from build123d import *

# Parameters (mm, degrees)
SKETCH1_R           = 10.75
BOSS_EXTRUDE1_DEPTH = 3
SKETCH2_R           = 10.75
BOSS_EXTRUDE2_DEPTH = 5.5
DRAFT5_START        = -9.337185289
DRAFT5_DEPTH        = 18.674370578
SKETCH3_W           = 5.126913696
SKETCH3_H           = 18.674370578
BOSS_EXTRUDE3_DEPTH = 17
CUT_EXTRUDE1_REACH  = 59.708
CUT_EXTRUDE2_REACH  = 59.708
SKETCH5_R           = 4


# Read off the part's stored shape, not the designer's step: Draft5
with BuildPart() as part:
    # Sketch1 → Boss-Extrude1 (new body)
    with BuildSketch(Plane(origin=(0, 0, 0), x_dir=(0, 0, -1), z_dir=(1, 0, 0))):
        with BuildLine():
            ThreePointArc((-4.479326664, 23.069148936), (0, -23.5), (4.479326664, 23.069148936))
            ThreePointArc((4.479326664, 23.069148936), (0, 19), (-4.479326664, 23.069148936))
        make_face()
        Circle(SKETCH1_R, mode=Mode.SUBTRACT)
    extrude(amount=BOSS_EXTRUDE1_DEPTH)

    # Sketch2 → Boss-Extrude2 (add)
    # profile 1 of 7: a face of its own
    with BuildSketch(Plane(origin=(3, 0, 0), x_dir=(0, 0, -1), z_dir=(1, 0, 0))):
        with BuildLine():
            Line((-15.626913696, -9.337185289), (-15.626913696, 9.337185289))
            Line((-15.626913696, 9.337185289), (-21.565411447, 9.337185289))
            ThreePointArc((-21.565411447, 9.337185289), (-22.146716975, 7.859575512), (-22.626913696, 6.346083564))
            Line((-22.626913696, 6.346083564), (-22.626913696, -6.346083564))
            ThreePointArc((-22.626913696, -6.346083564), (-22.146716975, -7.859575512), (-21.565411447, -9.337185289))
            Line((-21.565411447, -9.337185289), (-15.626913696, -9.337185289))
        make_face()
    # profile 2 of 7: a face of its own
    with BuildSketch(Plane(origin=(3, 0, 0), x_dir=(0, 0, -1), z_dir=(1, 0, 0))):
        Polygon((-15.626913696, -9.337185289), (-15.626913696, 9.337185289), (-8.736803998, 14.760144229), (8.736803998, 14.760144229), (15.626913696, 9.337185289), (15.626913696, -9.337185289), (8.736803998, -14.760144229), (-8.736803998, -14.760144229), align=None)
        Circle(SKETCH2_R, mode=Mode.SUBTRACT)
    # profile 3 of 7: a face of its own
    with BuildSketch(Plane(origin=(3, 0, 0), x_dir=(0, 0, -1), z_dir=(1, 0, 0))):
        with BuildLine():
            Line((21.565411447, 9.337185289), (15.626913696, 9.337185289))
            Line((15.626913696, 9.337185289), (15.626913696, -9.337185289))
            Line((15.626913696, -9.337185289), (21.565411447, -9.337185289))
            ThreePointArc((21.565411447, -9.337185289), (22.146716975, -7.859575512), (22.626913696, -6.346083564))
            Line((22.626913696, -6.346083564), (22.626913696, 6.346083564))
            ThreePointArc((22.626913696, 6.346083564), (22.146716975, 7.859575512), (21.565411447, 9.337185289))
        make_face()
    # profile 4 of 7: a face of its own
    with BuildSketch(Plane(origin=(3, 0, 0), x_dir=(0, 0, -1), z_dir=(1, 0, 0))):
        with BuildLine():
            ThreePointArc((-22.626913696, 6.346083564), (-22.146716975, 7.859575512), (-21.565411447, 9.337185289))
            Line((-21.565411447, 9.337185289), (-22.626913696, 9.337185289))
            Line((-22.626913696, 9.337185289), (-22.626913696, 6.346083564))
        make_face()
    # profile 5 of 7: a face of its own
    with BuildSketch(Plane(origin=(3, 0, 0), x_dir=(0, 0, -1), z_dir=(1, 0, 0))):
        with BuildLine():
            Line((-22.626913696, -9.337185289), (-21.565411447, -9.337185289))
            ThreePointArc((-21.565411447, -9.337185289), (-22.146716975, -7.859575512), (-22.626913696, -6.346083564))
            Line((-22.626913696, -6.346083564), (-22.626913696, -9.337185289))
        make_face()
    # profile 6 of 7: a face of its own
    with BuildSketch(Plane(origin=(3, 0, 0), x_dir=(0, 0, -1), z_dir=(1, 0, 0))):
        with BuildLine():
            Line((22.626913696, 9.337185289), (21.565411447, 9.337185289))
            ThreePointArc((21.565411447, 9.337185289), (22.146716975, 7.859575512), (22.626913696, 6.346083564))
            Line((22.626913696, 6.346083564), (22.626913696, 9.337185289))
        make_face()
    # profile 7 of 7: a face of its own
    with BuildSketch(Plane(origin=(3, 0, 0), x_dir=(0, 0, -1), z_dir=(1, 0, 0))):
        with BuildLine():
            ThreePointArc((22.626913696, -6.346083564), (22.146716975, -7.859575512), (21.565411447, -9.337185289))
            Line((21.565411447, -9.337185289), (22.626913696, -9.337185289))
            Line((22.626913696, -9.337185289), (22.626913696, -6.346083564))
        make_face()
    extrude(amount=BOSS_EXTRUDE2_DEPTH)

    # Draft5 outline → Draft5 (cut)
    with BuildSketch(Plane(origin=(0, 0, 0), x_dir=(1, 0, 0), z_dir=(0, 1, 0)).offset(DRAFT5_START)):
        Polygon((3, 22.626913696), (3, 21.153193137), (8.5, 22.626913696), align=None)
        Polygon((3, -21.153193137), (3, -22.626913696), (8.5, -22.626913696), align=None)
    extrude(amount=DRAFT5_DEPTH, mode=Mode.SUBTRACT)

    # Sketch3 → Boss-Extrude3 (add)
    with BuildSketch(Plane(origin=(8.5, 0, 0), x_dir=(0, 0, -1), z_dir=(1, 0, 0))):
        with Locations((-20.063456848, 0)):
            Rectangle(SKETCH3_W, SKETCH3_H)
        with Locations((20.063456848, 0)):
            Rectangle(SKETCH3_W, SKETCH3_H)
    extrude(amount=BOSS_EXTRUDE3_DEPTH)

    # Cut-Extrude1: up to this face of the body (flat: up to its plane)
    cut_extrude1_end = Plane(part.part.faces().sort_by_distance((17, 0, -22.626913696))[0])
    # Sketch4 → Cut-Extrude1 (cut, up to the picked face)
    with BuildSketch(Plane.XY.offset(22.626913696), mode=Mode.PRIVATE) as cut_extrude1_sk1:
        with BuildLine():
            Line((17, 9.337185289), (17, 12.880835783))
            Line((17, 12.880835783), (29.443712865, 12.880835783))
            Line((29.443712865, 12.880835783), (29.443712865, -13.088571654))
            Line((29.443712865, -13.088571654), (17, -13.088571654))
            Line((17, -13.088571654), (17, -9.337185289))
            ThreePointArc((17, -9.337185289), (25.5, 0), (17, 9.337185289))
        make_face()
    cut_extrude1_tool1 = split(extrude(cut_extrude1_sk1.sketch, amount=-CUT_EXTRUDE1_REACH, mode=Mode.PRIVATE), bisect_by=cut_extrude1_end, keep=Keep.BOTH, mode=Mode.PRIVATE)
    add(cut_extrude1_tool1.solids().sort_by(Axis((17.287968, 11.109011, 22.626914), (0, 0, -1)))[0], mode=Mode.SUBTRACT)

    # Cut-Extrude2: up to this face of the body (flat: up to its plane)
    cut_extrude2_end = Plane(part.part.faces().sort_by_distance((16.148390538, 0, -22.626913696))[0])
    # Sketch5 → Cut-Extrude2 (cut, up to the picked face)
    with BuildSketch(Plane.XY.offset(22.626913696), mode=Mode.PRIVATE) as cut_extrude2_sk1:
        with Locations(Location((18.5, 0, 0), (0, 0, 270))):
            Circle(SKETCH5_R)
    cut_extrude2_tool1 = split(extrude(cut_extrude2_sk1.sketch, amount=-CUT_EXTRUDE2_REACH, mode=Mode.PRIVATE), bisect_by=cut_extrude2_end, keep=Keep.BOTH, mode=Mode.PRIVATE)
    add(cut_extrude2_tool1.solids().sort_by(Axis((18.5, 0, 22.626914), (0, 0, -1)))[0], mode=Mode.SUBTRACT)


solid = part.part
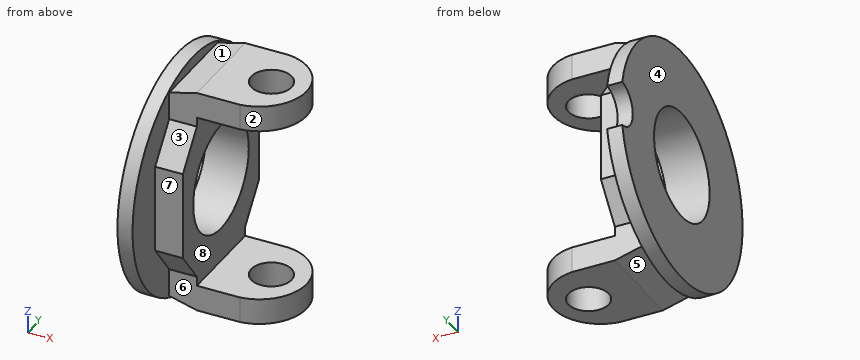
Could you check a few things on this model? Use its own coordinates, in mm. Face numbers are marked on the shaded views. A direction names the side the tool comes from. Give positions to 0.01 mm unless a question says otherwise; leave off trailing zeros. Loops run counter-clockwise (first coordinate to the right, second up) from the corner with the lowest first, then second, coordinate; pieces in that order, holes last. Notation, with made-up numbers: (17.25, 77) -> (47.25, 77) arc R21 cw to (47.25, 90) -> close; hole circle Ø2 at (81, 14). An arc over 180 degrees is marked (long way). Return JSON: item names as keys, results as strings.
Item 1: If we section it at B-B on y = 0: List the corners of the cut face in (x, z) for me, plus the area to 3 significant figures.
Geometry results:
{"outline": "(0, -23.5) -> (3, -23.5) -> (3, -21.15) -> (8.5, -22.63) -> (14.5, -22.63) -> (14.5, -17.5) -> (8.5, -17.5) -> (8.5, -10.75) -> (0, -10.75) -> close; (0, 10.75) -> (8.5, 10.75) -> (8.5, 17.5) -> (14.5, 17.5) -> (14.5, 22.63) -> (8.5, 22.63) -> (3, 21.15) -> (3, 23.5) -> (0, 23.5) -> close; (22.5, -22.63) -> (25.5, -22.63) -> (25.5, -17.5) -> (22.5, -17.5) -> close; (22.5, 17.5) -> (25.5, 17.5) -> (25.5, 22.63) -> (22.5, 22.63) -> close", "area": "291 mm²"}
Item 2: I'm going to push flat-ended pins straight in: pin 1 (7.5 mm diameter, centred on x = 9.5, z = 20, fed in from +Y); pin 2 (4 mm diameter, centred on y = -12, z = -14.5, fed in from -X); pin 3 (1.6 mm diameter, centred on x = 5, z = -4.5, fed in from -Y); pin 4 (6 mm diameter, centred on x = 6.5, z = -4, fed in from +Y). Where does each tip first touch, or does it pass through?
Geometry results:
{"pin 1": "stops at y = 9.34", "pin 2": "stops at x = 0", "pin 3": "stops at y = -14.76", "pin 4": "stops at y = 14.76"}
Item 3: If we section it at A-A on z = 0: List the corners of the cut face in (x, y) for me, plus the area to 3 significant figures.
Geometry results:
{"outline": "(0, -23.5) -> (3, -23.5) -> (3, -14.76) -> (8.5, -14.76) -> (8.5, -10.75) -> (0, -10.75) -> close; (0, 10.75) -> (8.5, 10.75) -> (8.5, 14.76) -> (3, 14.76) -> (3, 19) -> (0, 19) -> close", "area": "107 mm²"}
Item 4: If we section it at C-C on x = 18.5: List the corners of the cut face in (y, z) for me, plus the area to 3 significant figures.
Geometry results:
{"outline": "(-9.07, -22.63) -> (-4, -22.63) -> (-4, -17.5) -> (-9.07, -17.5) -> close; (-9.07, 17.5) -> (-4, 17.5) -> (-4, 22.63) -> (-9.07, 22.63) -> close; (4, -22.63) -> (9.07, -22.63) -> (9.07, -17.5) -> (4, -17.5) -> close; (4, 17.5) -> (9.07, 17.5) -> (9.07, 22.63) -> (4, 22.63) -> close", "area": "104 mm²"}
Item 5: If we section it at D-D on y = 6.5: List the corners of the cut face in (x, z) for me, plus the area to 3 significant figures.
Geometry results:
{"outline": "(0, -22.58) -> (3, -22.58) -> (3, -21.15) -> (8.5, -22.63) -> (22.88, -22.63) -> (22.88, -17.5) -> (8.5, -17.5) -> (8.5, -8.56) -> (0, -8.56) -> close; (0, 8.56) -> (8.5, 8.56) -> (8.5, 17.5) -> (22.88, 17.5) -> (22.88, 22.63) -> (8.5, 22.63) -> (3, 21.15) -> (3, 22.58) -> (0, 22.58) -> close", "area": "378 mm²"}
Item 6: We'd pull the mould along X, two halves only. Please class the marked faces 1, 2, 3 and 4: +X half, -X half, draft (parallel to the pull), parting line (faces both ways), or undercut.
Geometry results:
{"face 1": "undercut", "face 2": "+X half", "face 3": "draft", "face 4": "-X half"}
Item 7: Which directions (+Z, -Z, +X, -X, +Y, -Y) give clear straight access to the entire face, cutting with the end or side of a thin tool? Please do the marked faces 5, 6, 7 and 8.
Geometry results:
{"face 5": "-Z, +Y, -Y", "face 6": "-Z, +X, -Y", "face 7": "+Z, -Z, +X, -Y", "face 8": "+X, +Y, -Y"}
Item 8: I need wall thicknesses on L1, parallel to Y at x = 5, z = 0; L2, parallel to X at y = 0, z = -19.3; L3, parallel to Y at x = 2.5, z = 0. Which ranges of each line are inside material? Lowest first, please. Write a range as from..to.
Geometry results:
{"L1": "y = -14.76..-10.75, 10.75..14.76", "L2": "x = 0..14.5, 22.5..25.5", "L3": "y = -23.5..-10.75, 10.75..19"}
